```python
from build123d import *
from build123d import SkipClean  # not in build123d's __all__

# Parameters (mm, degrees)
F0_R      = 6.35
F1_DEPTH  = 47.625
F5_R      = 14.8376639977
F6_DEPTH  = 48.26
F7_R      = 10.16
F8_DEPTH  = 25.4
F10_R     = 4.7625
F11_DEPTH = 127
F9_R      = 2.286
F12_DEPTH = 44.083008926


with BuildPart() as f1:
    # F0 (on Top) → F1 (new body)
    with BuildSketch(Plane.XY):
        Polygon((0, 47.625), (0, 0), (40.767, 0), (40.767, 8.89), (59.817, 8.89), (59.817, 0), (90.297, 0), (90.297, 47.625), align=None)
        with Locations((12.7, 12.7)):
            Circle(F0_R, mode=Mode.SUBTRACT)
        with Locations((12.7, 34.925)):
            Circle(F0_R, mode=Mode.SUBTRACT)
    extrude(amount=F1_DEPTH)

    # F3 (on offset) → F4 (revolve, cut)
    with BuildSketch(Plane(origin=(0, 0, 23.8125), x_dir=(1, 0, 0), z_dir=(0, 0, -1))):
        with BuildLine():
            Line((90.297, -35.2425), (90.297, -12.3825))
            ThreePointArc((90.297, -12.3825), (78.867, -23.8125), (90.297, -35.2425))
        make_face()
    with SkipClean():  # cleaning this boolean's faces spoils the solid; the shape is the same uncleaned
        revolve(axis=Axis((90.297, 23.8125, 23.8125), (0, 1, 0)), mode=Mode.SUBTRACT)

    # F5 (on face) → F6 (join)
    with BuildSketch(Plane(origin=(0, 0, 0), x_dir=(0, -1, 0), z_dir=(-1, 0, 0))):
        with Locations((-23.8125, 23.8125)):
            Circle(F5_R)
    with SkipClean():  # cleaning this boolean's faces spoils the solid; the shape is the same uncleaned
        extrude(amount=F6_DEPTH)

    # F7 (on face) → F8 (join)
    with BuildSketch(Plane(origin=(-48.26, 0, 0), x_dir=(0, -1, 0), z_dir=(-1, 0, 0))):
        with Locations((-23.8125, 23.8125)):
            Circle(F7_R)
    with SkipClean():  # cleaning this boolean's faces spoils the solid; the shape is the same uncleaned
        extrude(amount=F8_DEPTH)

    # F10 (on Front) → F11 (cut)
    with BuildSketch(Plane.XZ):
        with Locations((-25.4, 23.8125)):
            Circle(F10_R)
    with SkipClean():  # cleaning this boolean's faces spoils the solid; the shape is the same uncleaned
        extrude(amount=-F11_DEPTH, mode=Mode.SUBTRACT)

    # F9 (on face) → F12 (cut, through all)
    with BuildSketch(Plane(origin=(-73.66, 0, 0), x_dir=(0, -1, 0), z_dir=(-1, 0, 0))):
        with Locations((-23.8125, 23.8125)):
            Circle(F9_R)
    with SkipClean():  # cleaning this boolean's faces spoils the solid; the shape is the same uncleaned
        extrude(amount=-F12_DEPTH, mode=Mode.SUBTRACT)


solid = f1.part
```
For this review, take the finished solid that the model builds, in its own axes (mm). A direction names the side the tool comes from. Round coordinates to 2 decimals unless told otherwise and drop trailing zeros. Write each loop counter-clockwise with the first axis right and the second up, starting at its lowest first coordinate (ties: lowest second). Pieces come first, ordered by that corner, then holes. Notation, with made-up numbers: (6, 38.25) -> (38, 38.25) arc R37 ccw to (38, 76.25) -> close; hole circle Ø4 at (-4.75, -25.5). An arc over 180 degrees is marked (long way). Use one line per item in the form item = value.
1) Tool access review of faces 1 (the flat face through (-73.66, 22, 22)), 2 (the cylindrical face through (-51.93, 21.7, 22.94)), 3 (the flat face through (40.767, 4, 23)): name each direction out of +Z, -Z, +X, -X, +Y, -Y from which nothing blocks a thin tool from reaching the whole face with its end or side.
Found:
face_1 = +Z, -Z, -X, +Y, -Y
face_2 = -X
face_3 = +Z, -Z, -Y
2) Take a section at D-D, the plane z = 37. Write out the cut boundary in (x, y) (3 decimals), and give its area (3 significant figures).
Found:
outline = (-48.26, 17.012) -> (0, 17.012) -> (0, 0) -> (40.767, 0) -> (40.767, 8.89) -> (59.817, 8.89) -> (59.817, 0) -> (90.297, 0) -> (90.297, 47.625) -> (0, 47.625) -> (0, 30.613) -> (-48.26, 30.613) -> close; hole circle Ø12.7 at (12.7, 12.7); hole circle Ø12.7 at (12.7, 34.925)
area = 4,530 mm2
3) Take a section at A-A, the plane x = 12.7. Write out the cut boundary in (y, z) (3 decimals), and give its area (3 significant figures).
Found:
outline = (0, 0) -> (6.35, 0) -> (6.35, 47.625) -> (0, 47.625) -> close; (19.05, 0) -> (28.575, 0) -> (28.575, 47.625) -> (19.05, 47.625) -> close; (41.275, 0) -> (47.625, 0) -> (47.625, 47.625) -> (41.275, 47.625) -> close
area = 1,060 mm2
4) Mouldability with a two-part tool opening along Z and no side actions: class faces 4 (the flat face through (45, 24, 47.625)), 5 (the cylindrical face through (-21, 23.6, 21.99)), 6 (the flat face through (90.297, 13, 18)) as +Z half, -Z half, draft (parallel to the pull), parting line (faces both ways), or undercut.
Found:
face_4 = +Z half
face_5 = undercut
face_6 = draft
5) Take a section at B-B, the plane z = 10.5. Write out the cut boundary in (x, y) (3 decimals).
Found:
outline = (-48.26, 17.26) -> (0, 17.26) -> (0, 0) -> (40.767, 0) -> (40.767, 8.89) -> (59.817, 8.89) -> (59.817, 0) -> (90.297, 0) -> (90.297, 47.625) -> (0, 47.625) -> (0, 30.365) -> (-48.26, 30.365) -> close; hole circle Ø12.7 at (12.7, 12.7); hole circle Ø12.7 at (12.7, 34.925)
6) To check wall thickness, follow L1, parallel to Y at x = 12.7, z = 17 (3 decimals); L2, parallel to Y at x = 16, z = 23.5 (3 decimals); L3, parallel to X at y = 38.5, z = 23. State the ranges of each line that lie inside material, in increasing order. Write a range as from..to.
Found:
L1 = 0..6.35, 19.05..28.575, 41.275..47.625
L2 = 0..7.275, 18.125..29.5, 40.35..47.625
L3 = -48.26..-30.09, -20.71..7.45, 17.95..90.3
7) Clearance check with flat-ended pins moving along their axes: pin 1 (8.5 mm diameter, centred on x = -25.4, z = 23.81, fed in from +Y); pin 2 (4.5 mm diameter, centred on y = 3, z = 22, fed in from -X); pin 3 (1.5 mm diameter, centred on x = -36.5, y = 20, fed in from -Z); pin 4 (8 mm diameter, centred on x = -16.5, z = 15, fed in from -Y). State where each tip first meets the part, or that it passes through.
Found:
pin_1 = through
pin_2 = 0
pin_3 = 9.29
pin_4 = 9.78
